from build123d import *

# Parameters (mm, degrees)
SKETCH1_W           = 120
SKETCH1_H           = 50
BOSS_EXTRUDE1_DEPTH = 3
SKETCH2_R           = 2.95
SKETCH2_R_2         = 2.3
SKETCH2_W           = 12.75
SKETCH2_H           = 18.4
CUT_EXTRUDE1_DEPTH  = 3
SKETCH3_W           = 8.9
SKETCH3_H           = 10.9
CUT_EXTRUDE2_DEPTH  = 10


with BuildPart() as part:
    # Sketch1 → Boss-Extrude1 (new body)
    with BuildSketch(Plane(origin=(0, 0, 0), x_dir=(1, 0, 0), z_dir=(0, 1, 0))):
        with Locations((-60, 25)):
            Rectangle(SKETCH1_W, SKETCH1_H)
    extrude(amount=BOSS_EXTRUDE1_DEPTH)

    # Sketch2 → Cut-Extrude1 (cut)
    with BuildSketch(Plane(origin=(0, 3, 0), x_dir=(1, 0, 0), z_dir=(0, 1, 0))):
        with Locations(Location((-60, 25, 0), (0, 0, 270))):  # turned: the seam where the file's is
            Circle(SKETCH2_R)
        with Locations(Location((-45, 25, 0), (0, 0, 270))):  # turned: the seam where the file's is
            Circle(SKETCH2_R_2)
        with Locations(Location((-30, 25, 0), (0, 0, 270))):  # turned: the seam where the file's is
            Circle(SKETCH2_R_2)
        with Locations((-100, 25)):
            Rectangle(SKETCH2_W, SKETCH2_H)
    extrude(amount=-CUT_EXTRUDE1_DEPTH, mode=Mode.SUBTRACT)

    # Sketch3 → Cut-Extrude2 (cut)
    with BuildSketch(Plane(origin=(0, 3, 0), x_dir=(1, 0, 0), z_dir=(0, 1, 0))):
        with Locations((-81.74741462, 25.690314881)):
            Rectangle(SKETCH3_W, SKETCH3_H)
    extrude(amount=-CUT_EXTRUDE2_DEPTH, mode=Mode.SUBTRACT)


solid = part.part
Model file for the job. Use its own axes, mm. A direction names the side the tool comes from. Coordinates: 2 decimals unless noted, no trailing zeros. Write each loop counter-clockwise with the first axis right and the second up, starting at its lowest first coordinate (ties: lowest second). Pieces come first, ordered by that corner, then holes. Notation, with made-up numbers: (74.25, 18) -> (92.25, 18) arc R30 ccw to (92.25, 52) -> close; hole circle Ø5 at (6.25, 55). An arc over 180 degrees is marked (long way). One line per item, written item: value. Start each with the question number.
1) Probe probe 1 along X at (y, z) = (0.8, -25) (3 decimals); probe 2 along X at (y, z) = (2.45, -28.5) (3 decimals); probe 3 along Z at (x, y) = (-103, 0.25). List the from-to ranges inside material, lowest first.
2) Flat gauge pin, fed straight in: pin 1 Ø0.9 at (x, y) = (-82, 2) entering from +Z. Where does the tip first touch, or does it go through?
3) Pull direction X, two halves, no side cores. Call faces 3 (the face through (-61, 1, 0)), 4 (the face through (0, 1, -25)), 5 (the face through (-93.625, 2, -25)): +X half, -X half, draft (parallel to the pull), parting line (faces both ways), or undercut.
4) Slice it at B-B on z = -17. Write the cut outline in (x, y) (3 decimals), then the cut area to 3 significant figures.
5) Slice it at A-A on x = -45. Write the cut outline in (y, z).
6) Slice it at C-C on z = -25. Write the cut outline in (x, y) (3 decimals).
7) Which spindle directions (+Z, -Z, +X, -X, +Y, -Y) get a long thin tool onto all of the face, cutting with end or side? Do faces 1 (the face through (-61, 1, -50)), 2 (the face through (-106.375, 2, -25)). Say none if no direction does.
8) Slice it at D-D on y = 2.45. Write the cut outline in (x, z) (3 decimals).
Answers follow:
1. probe 1: -120 to -106.375, -93.625 to -86.197, -77.297 to -62.95, -57.05 to -47.3, -42.7 to -32.3, -27.7 to 0
1. probe 2: -120 to -106.375, -93.625 to -86.197, -77.297 to 0
1. probe 3: -50 to -34.2, -15.8 to 0
2. pin 1: z = 0
3. face 3: draft
3. face 4: +X half
3. face 5: undercut
4. outline: (-120, 0) -> (-106.375, 0) -> (-106.375, 3) -> (-120, 3) -> close; (-93.625, 0) -> (0, 0) -> (0, 3) -> (-93.625, 3) -> close
4. area: 322 mm2
5. outline: (0, -50) -> (3, -50) -> (3, -27.3) -> (0, -27.3) -> close; (0, -22.7) -> (3, -22.7) -> (3, 0) -> (0, 0) -> close
6. outline: (-120, 0) -> (-106.375, 0) -> (-106.375, 3) -> (-120, 3) -> close; (-93.625, 0) -> (-86.197, 0) -> (-86.197, 3) -> (-93.625, 3) -> close; (-77.297, 0) -> (-62.95, 0) -> (-62.95, 3) -> (-77.297, 3) -> close; (-57.05, 0) -> (-47.3, 0) -> (-47.3, 3) -> (-57.05, 3) -> close; (-42.7, 0) -> (-32.3, 0) -> (-32.3, 3) -> (-42.7, 3) -> close; (-27.7, 0) -> (0, 0) -> (0, 3) -> (-27.7, 3) -> close
7. face 1: -Z, +X, -X, +Y, -Y
7. face 2: +Y, -Y
8. outline: (-120, -50) -> (0, -50) -> (0, 0) -> (-120, 0) -> close; hole (-106.375, -34.2) -> (-93.625, -34.2) -> (-93.625, -15.8) -> (-106.375, -15.8) -> close; hole (-86.197, -31.14) -> (-77.297, -31.14) -> (-77.297, -20.24) -> (-86.197, -20.24) -> close; hole circle Ø5.9 at (-60, -25); hole circle Ø4.6 at (-45, -25); hole circle Ø4.6 at (-30, -25)
